Check sheet for the drawn part. Datum: minimum x, y, z corner. Units: mm. Round coordinates to 2 decimals unless told otherwise and drop trailing zeros. Loops run counter-clockwise (first coordinate to the right, second up) from the corner with the lowest first, then second, coordinate; pieces in that order, holes last.
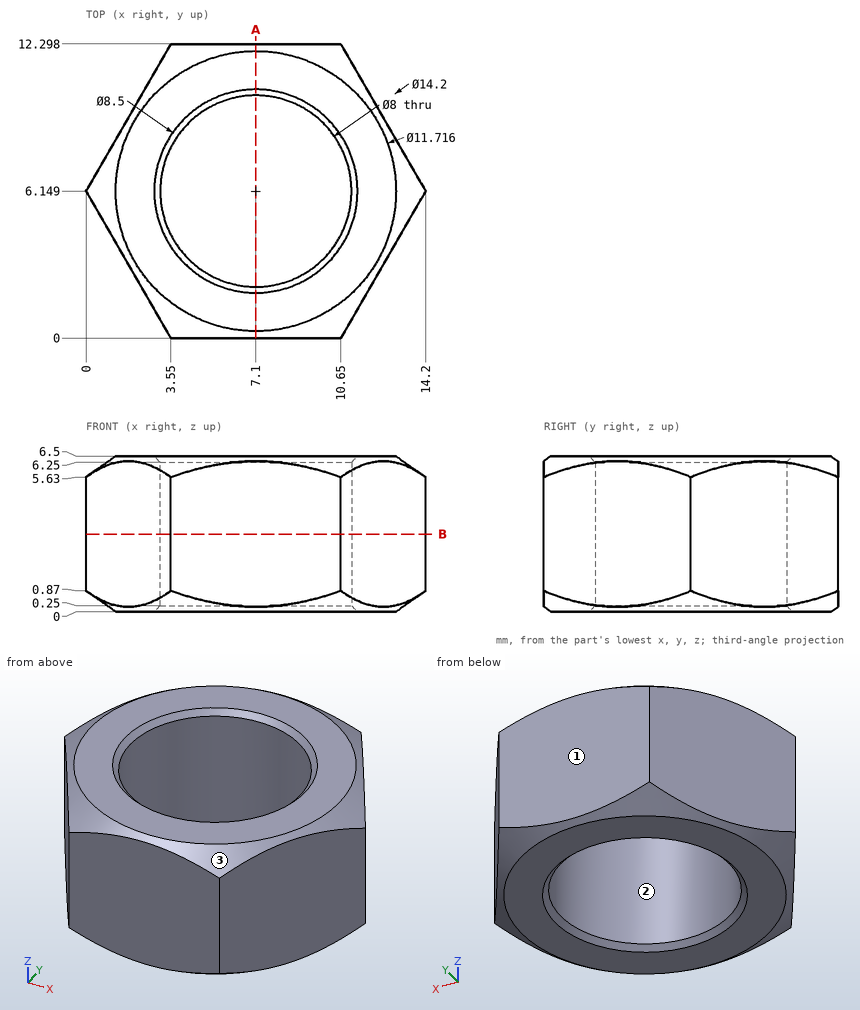
1) Mould release check, pull along Y, two halves, no side actions. Record for the marked faces 1, 2 and 3: +Y half, -Y half, draft (parallel to the pull), parting line (faces both ways), or undercut.
Report:
face 1: +Y half
face 2: undercut
face 3: parting line
2) Sectioned sample at B-B, the plane z = 3.25. Record the cut outline in (x, y).
Report:
outline: (0, 6.15) - (3.55, 0) - (10.65, 0) - (14.2, 6.15) - (10.65, 12.3) - (3.55, 12.3) - close; hole circle Ø8 at (7.1, 6.15)
3) Scan lines: line 1 along Y through (x, z) = (7.1, 4.85); line 2 along X through (y, z) = (4.5, 4) (1 decimal); line 3 along Y through (x, z) = (9.75, 5.75) (1 decimal). Record each from-to range of solid material in increasing order.
Report:
line 1: y = 0 to 2.15, 10.15 to 12.3
line 2: x = 1 to 3.5, 10.7 to 13.2
line 3: y = 0 to 3.2, 9.1 to 12.3
4) Sectioned sample at A-A, the plane x = 7.1. Record the cut outline in (y, z).
Report:
outline: (0, 0.2) - (0.29, 0) - (1.9, 0) - (2.15, 0.25) - (2.15, 6.25) - (1.9, 6.5) - (0.29, 6.5) - (0, 6.3) - close; (10.15, 0.25) - (10.4, 0) - (12.01, 0) - (12.3, 0.2) - (12.3, 6.3) - (12.01, 6.5) - (10.4, 6.5) - (10.15, 6.25) - close
5) Gauge pin test, flat ends, axial feed: pin 1 (1.5 mm diameter, centred on x = 10, y = 6, fed in from -Z); pin 2 (3 mm diameter, centred on y = 2, z = 5, fed in from +X). Record the tip position at first contact, or that the pin passes through.
Report:
pin 1: passes through
pin 2: stops at x = 12.67
